The listing builds one solid part. Answer for the finished solid, in the listing's coordinates (mm). A direction names the side the tool comes from. Coordinates: 2 decimals unless noted, no trailing zeros. Order: outer loops, then holes, each group sorted by start corner. A loop starts at its lowest first (then second) coordinate and runs counter-clockwise, first axis right, second up.
from build123d import *

# Parameters (mm, degrees)
SKETCH1_W                      = 32.5
SKETCH1_H                      = 80.25
BOSS_EXTRUDE1_DEPTH            = 6
BOSS_EXTRUDE2_DEPTH            = 11
F_6_0MM_DOWEL_HOLE1_D          = 6
M5X0_8_TAPPED_HOLE1_D          = 4.2
CBORE_FOR_M3_SHCS1_D           = 3.4
CBORE_FOR_M3_SHCS1_CBORE_D     = 6.5
CBORE_FOR_M3_SHCS1_CBORE_DEPTH = 3
F_1_0_1_DIAMETER_HOLE1_D       = 1
SKETCH12_R                     = 1.5
CUT_EXTRUDE1_DEPTH             = 5
SKETCH13_W                     = 6
SKETCH13_H                     = 35
CUT_EXTRUDE2_DEPTH             = 84.624906577
FILLET1_R                      = 2.38125
SKETCH14_W                     = 34.5
SKETCH14_H                     = 82.25
CUT_EXTRUDE3_DEPTH             = 84.624906577


with BuildPart() as part:
    # Sketch1 → Boss-Extrude1 (new body)
    with BuildSketch(Plane(origin=(0, 0, 0), x_dir=(1, 0, 0), z_dir=(0, 1, 0))):
        with Locations((0, -40.125)):
            Rectangle(SKETCH1_W, SKETCH1_H)
    extrude(amount=-BOSS_EXTRUDE1_DEPTH)

    # Sketch2 → Boss-Extrude2 (add)
    with BuildSketch(Plane(origin=(0, 0, 0), x_dir=(1, 0, 0), z_dir=(0, 1, 0))):
        with BuildLine():
            Line((-5.032198748, 0), (5.032198748, 0))
            ThreePointArc((5.032198748, 0), (1.230950737, -23.858861929), (16.25, -42.782998323))
            Line((16.25, -42.782998323), (16.25, -80.25))
            Line((16.25, -80.25), (-16.25, -80.25))
            Line((-16.25, -80.25), (-16.25, -42.782998323))
            ThreePointArc((-16.25, -42.782998323), (-1.230950737, -23.858861929), (-5.032198748, 0))
        make_face()
    extrude(amount=BOSS_EXTRUDE2_DEPTH)

    # Ø6.0mm Dowel Hole1 (through all)
    with Locations(Plane(origin=(16.25, 0, 0), x_dir=(0, 0, -1), z_dir=(1, 0, 0))):
        with Locations((-73.25, 6), (-55.25, 6)):
            Hole(F_6_0MM_DOWEL_HOLE1_D / 2)

    # M5x0.8 Tapped Hole1 (through all)
    with Locations(Plane(origin=(16.25, 0, 0), x_dir=(0, 0, -1), z_dir=(1, 0, 0))):
        with Locations((-64.25, 6)):
            Hole(M5X0_8_TAPPED_HOLE1_D / 2)

    # CBORE for M3 SHCS1 (through all)
    with Locations(Plane(origin=(0, 0, 0), x_dir=(1, 0, 0), z_dir=(0, 1, 0))):
        with Locations((-11, -5.25), (11, -5.25), (11, -27.25), (-11, -27.25)):
            CounterBoreHole(CBORE_FOR_M3_SHCS1_D / 2, CBORE_FOR_M3_SHCS1_CBORE_D / 2, CBORE_FOR_M3_SHCS1_CBORE_DEPTH)

    # Ø1.0 (1) Diameter Hole1 (through all)
    with Locations(Plane(origin=(0, 11, 0), x_dir=(1, 0, 0), z_dir=(0, 1, 0))):
        with Locations((0, -16.25)):
            Hole(F_1_0_1_DIAMETER_HOLE1_D / 2)

    # Sketch12 → Cut-Extrude1 (cut)
    with BuildSketch(Plane.XZ.offset(6)):
        with Locations(Location((0, 16.25, 0), (0, 0, 270))):
            Circle(SKETCH12_R)
    extrude(amount=-CUT_EXTRUDE1_DEPTH, mode=Mode.SUBTRACT)

    # Sketch13 → Cut-Extrude2 (cut, through all)
    with BuildSketch(Plane(origin=(0, 11, 0), x_dir=(1, 0, 0), z_dir=(0, 1, 0))):
        with Locations((-13.25, -62.75)):
            Rectangle(SKETCH13_W, SKETCH13_H)
        with Locations((13.25, -62.75)):
            Rectangle(SKETCH13_W, SKETCH13_H)
    extrude(amount=-CUT_EXTRUDE2_DEPTH, mode=Mode.SUBTRACT)

    # Fillet1
    fillet1_edges = [part.edges().sort_by_distance(p)[0] for p in [
        (-10.25, 2.5, 45.25),
        (10.25, 2.5, 45.25),
    ]]
    fillet(fillet1_edges, radius=FILLET1_R)

    # Sketch14 → Cut-Extrude3 (cut, through all)
    with BuildSketch(Plane(origin=(0, 11, 0), x_dir=(1, 0, 0), z_dir=(0, 1, 0))):
        with Locations((0, -40.125)):
            Rectangle(SKETCH14_W, SKETCH14_H)
        with BuildLine():
            Line((-10, -80.25), (-10, -36.41515139))
            ThreePointArc((-10, -36.41515139), (-10.816699867, -33.676538602), (-13, -31.832575695))
            ThreePointArc((-13, -31.832575695), (-15.183300133, -29.988612788), (-16, -27.25))
            Line((-16, -27.25), (-16, -5.25))
            ThreePointArc((-16, -5.25), (-14.535533906, -1.714466094), (-11, -0.25))
            Line((-11, -0.25), (11, -0.25))
            ThreePointArc((11, -0.25), (14.535533906, -1.714466094), (16, -5.25))
            Line((16, -5.25), (16, -27.25))
            ThreePointArc((16, -27.25), (15.183300133, -29.988612788), (13, -31.832575695))
            ThreePointArc((13, -31.832575695), (10.816699867, -33.676538602), (10, -36.41515139))
            Line((10, -36.41515139), (10, -80.25))
            Line((10, -80.25), (-10, -80.25))
        make_face(mode=Mode.SUBTRACT)
    extrude(amount=-CUT_EXTRUDE3_DEPTH, mode=Mode.SUBTRACT)


solid = part.part
(1) A tool of negligible diameter and unlimited length cuts with its end or side. For faces 1 (the cylindrical face through (7.753, -1.479, 5.107)), 2 (the flat face through (-16, -3, 16)), 3 (the cylindrical face through (0.07, -3.54, 17.75)), 4 (the flat face through (-10, 3, 59)), 5 (the cylindrical face through (-1.457, 5.423, 7.826)), from which of +Z, -Z, +X, -X, +Y, -Y can it reach the whole face along a straight path? Write none if from no direction.
(2) Find section D-D on x = 4. Determine the outline of the cut face in (y, z).
(3) Find section B-B on z = 55.25. Determine the outline of the cut face in (x, y), then the cut area to 3 significant figures.
(4) The mould has two halves that part along Z. Classify faces 6 (the cylindrical face through (14.5, -2.96, 1.68)), 7 (the cylindrical face through (-11.914, -4.521, 25.817)), 8 (the flat face through (0, 2, 80.25)): pulls with the +Z half, pulls with the -Z half, needs draft (parallel to the pull), parting line crosses it, or undercut.
(5) Find section C-C on y = 1.25. Determine the outline of the cut face in (x, z), then the cut area to 3 significant figures.
(6) Find the intervals of material crossed by probe 1 along X at (y, z) = (-5, 27.25); probe 2 along Y at (x, z) = (-0.5, 55.25); probe 3 along X at (y, z) = (-2.05, 16.25), in increasing order.
(7) Given pin 1 Ø5 at (x, z) = (10.5, 5.5) entering from +Y; pin 2 Ø5 at (y, z) = (2, 60.5) entering from +X; pin 3 Ø1 at (y, z) = (6.5, 58.5) entering from -X, each flat-ended and moving along its own axis, determine where each tip first touches the part or whether it passes through.
(8) Find section A-A on y = 6. Determine the outline of the cut face in (x, z), then the cut area to 3 significant figures.
Resolved:
1. face 1: +Y
1. face 2: +Z, -Z, -X, +Y, -Y
1. face 3: -Y
1. face 4: +Z, -X, +Y, -Y
1. face 5: -X, +Y
2. outline: (-6, 0.25) - (11, 0.25) - (11, 1.73) - (0, 1.73) - (0, 30.77) - (11, 30.77) - (11, 80.25) - (-6, 80.25) - close; hole circle Ø6 at (6, 55.25); hole circle Ø6 at (6, 73.25); hole circle Ø4.2 at (6, 64.25)
3. outline: (-10, -6) - (10, -6) - (10, 3) - (-10, 3) - close; (-10, 9) - (10, 9) - (10, 11) - (-10, 11) - close
3. area: 220 mm2
4. face 6: pulls with the -Z half
4. face 7: undercut
4. face 8: pulls with the +Z half
5. outline: (-10, 38.38) arc R30 cw to (-0.25, 16.68) arc R0.5 cw to (0.25, 16.68) arc R30 cw to (10, 38.38) - (10, 80.25) - (-10, 80.25) - close; (-4.87, 0.25) - (4.87, 0.25) arc R30 cw to (0.25, 15.82) arc R0.5 cw to (-0.25, 15.82) arc R30 cw to start
5. area: 1,040 mm2
6. probe 1: x = -16 to -12.7, -9.3 to 9.3, 12.7 to 16
6. probe 2: y = -6 to 3, 9 to 11
6. probe 3: x = -16 to -1.5, 1.5 to 16
7. pin 1: stops at y = -3
7. pin 2: stops at x = 10
7. pin 3: stops at x = -10
8. outline: (-10, 38.38) arc R30 cw to (-0.25, 16.68) arc R0.5 cw to (0.25, 16.68) arc R30 cw to (10, 38.38) - (10, 52.25) - (-10, 52.25) - close; (-10, 58.25) - (10, 58.25) - (10, 62.15) - (-10, 62.15) - close; (-10, 66.35) - (10, 66.35) - (10, 70.25) - (-10, 70.25) - close; (-10, 76.25) - (10, 76.25) - (10, 80.25) - (-10, 80.25) - close; (-4.87, 0.25) - (4.87, 0.25) arc R30 cw to (0.25, 15.82) arc R0.5 cw to (-0.25, 15.82) arc R30 cw to start
8. area: 713 mm2
